Autodesk Inventor part; units mm, degrees
ref_plane "YZ Plane" through (0, 0, 0) normal (1, 0, 0) x (0, 1, 0)
ref_plane "XZ Plane" through (0, 0, 0) normal (0, 1, 0) x (-1, 0, 0)
ref_plane "XY Plane" through (0, 0, 0) normal (0, 0, 1) x (1, 0, 0)
sketch "Sketch1" plane through (0, 0, 0) normal (0, 1, 0) x (-1, 0, 0)
  line L0 (0, 0) -> (25.4, 0)
  line L1 (25.4, 0) -> (25.4, -25.4)
  line L2 (25.4, -25.4) -> (0, -25.4)
  line L3 (0, -25.4) -> (0, 0)
  line L4 (23.4, -23.4) -> (23.4, -2)
  line L5 (23.4, -2) -> (2, -2)
  line L6 (2, -2) -> (2, -23.4)
  line L7 (2, -23.4) -> (23.4, -23.4)
  dimension "d0" = 25.4
  dimension "d1" = 25.4
  dimension "d2" = 2
extrude "Extrusion1" add sketch "Sketch1" along normal blind 152.4
sketch "Sketch2" plane through (-25.4, 0, 0) normal (0, 0, 1) x (1, 0, 0)
  line L0 (25.4, 0) -> (0, 0)
  circle A0 centre (12.7, 5.4) radius 2
  dimension "d6" = 4
extrude "Extrusion2" cut sketch "Sketch2" against normal through all
sketch "Sketch3" plane through (0, 0, 0) normal (1, 0, 0) x (0, 0, -1)
  line L0 (0, 0) -> (25.4, 0)
  circle A0 centre (12.7, 15.4) radius 2
  dimension "d10" = 4
extrude "Extrusion3" cut sketch "Sketch3" against normal through all
properties part number "Metal_Bone"
Read the model definition and answer for the solid it produces. Units are mm, in the model's axes. A direction names the side the tool comes from. Give positions to 0.01 mm unless a question says otherwise; leave off trailing zeros. Write each loop counter-clockwise with the first axis right and the second up, starting at its lowest first coordinate (ties: lowest second). Pieces come first, ordered by that corner, then holes. Notation, with made-up numbers: (-39.75, 60) -> (-1.75, 60) arc R17 ccw to (-1.75, 79) -> close; hole circle Ø10 at (75.25, 8). An arc over 180 degrees is marked (long way). Answer in a Markdown table with one row per item.
1) Each of these flat-tipped pins is pushed along its axis until it touches: pin 1 Ø4.5 at (y, z) = (15.4, -12.7) entering from +X; pin 2 Ø1 at (x, z) = (-3.5, -5.5) entering from -Y. Where does it stop, or does it pass through?
Results list:
| item | result |
|---|---|
| pin 1 | x = 0 |
| pin 2 | through |
2) Section C-C on y = 15.4 is taken. Give the vertices of the cut face in (x, z), plus the area to 3 significant figures.
Results list:
| item | result |
|---|---|
| outline | (-25.4, -25.4) -> (0, -25.4) -> (0, -14.7) -> (-2, -14.7) -> (-2, -23.4) -> (-23.4, -23.4) -> (-23.4, -14.7) -> (-25.4, -14.7) -> close; (-25.4, -10.7) -> (-23.4, -10.7) -> (-23.4, -2) -> (-2, -2) -> (-2, -10.7) -> (0, -10.7) -> (0, 0) -> (-25.4, 0) -> close |
| area | 171 mm^2 |
3) A tool of negligible diameter and unlimited length cuts with its end or side. For faces 4 (the flat face through (-13, 75, 0)), 5 (the flat face through (-23.4, 75, -13)), from which of +Z, -Z, +X, -X, +Y, -Y can it reach the whole face along a straight path? Write none if from no direction.
Results list:
| item | result |
|---|---|
| face 4 | +Z, +X, -X, +Y, -Y |
| face 5 | +Y, -Y |
4) Section B-B on z = -12.7 is taken. Give the vertices of the cut face in (x, y).
Results list:
| item | result |
|---|---|
| outline | (-25.4, 0) -> (-23.4, 0) -> (-23.4, 13.4) -> (-25.4, 13.4) -> close; (-25.4, 17.4) -> (-23.4, 17.4) -> (-23.4, 152.4) -> (-25.4, 152.4) -> close; (-2, 0) -> (0, 0) -> (0, 13.4) -> (-2, 13.4) -> close; (-2, 17.4) -> (0, 17.4) -> (0, 152.4) -> (-2, 152.4) -> close |
5) Determine the mould class of faces 1 (the flat face through (-13, 75, -25.4)), 2 (the cylindrical face through (-0.986, 17.086, -13.775)), 3 (the flat face through (0, 75, -13)) for opening direction Z: released by +Z, released by -Z, zero draft, split by the parting line, or undercut.
Results list:
| item | result |
|---|---|
| face 1 | released by -Z |
| face 2 | undercut |
| face 3 | zero draft |
6) Section D-D on y = 65.5 is taken. Give the vertices of the cut face in (x, z).
Results list:
| item | result |
|---|---|
| outline | (-25.4, -25.4) -> (0, -25.4) -> (0, 0) -> (-25.4, 0) -> close; hole (-23.4, -23.4) -> (-2, -23.4) -> (-2, -2) -> (-23.4, -2) -> close |
7) Section A-A on x = -18 is taken. Give the vertices of the cut face in (y, z), plus the area to 3 significant figures.
Results list:
| item | result |
|---|---|
| outline | (0, -25.4) -> (152.4, -25.4) -> (152.4, -23.4) -> (0, -23.4) -> close; (0, -2) -> (152.4, -2) -> (152.4, 0) -> (0, 0) -> close |
| area | 610 mm^2 |
8) Straight lines are drawn through the part: line 1 (Z direction, x = -13.75, y = 123); line 2 (Y direction, x = -23.9, z = -12.7). For each, find the intervals that lie inside material, in ascending order. Write a range as [from, to].
Results list:
| item | result |
|---|---|
| line 1 | [-25.4, -23.4], [-2, 0] |
| line 2 | [0, 13.4], [17.4, 152.4] |
